Could you check a few things on this model? Use its own coordinates, in mm. A direction names the side the tool comes from. Coordinates: 2 decimals unless noted, no trailing zeros. Loops run counter-clockwise (first coordinate to the right, second up) from the corner with the lowest first, then second, coordinate; pieces in that order, holes last. Notation, with made-up numbers: (85.25, 44.5) - (95.25, 44.5) arc R28 ccw to (95.25, 80.5) - close; hole circle Ø10 at (86.5, 54). An arc over 180 degrees is marked (long way). One line per item, written item: value. Start each with the question number.
(1) On a 3-axis mill with a long thin cutter (end or side, diameter ignored), from which of +Z, -Z, +X, -X, +Y, -Y can I reach the whole of each face in a straight line? I mean faces 4 (the face through (-12, 2, 16)), 5 (the face through (-12, -2, 8.271)), 6 (the face through (-13.5, -38.1, 13.662)), 7 (the face through (-17, -4.65, 12)), 8 (the face through (-17, 5, 13.662)). Say none if no direction works.
(2) If we section it at D-D on x = -15.75: Write out the boundary of the cut face in (y, z) (3 decimals), then the cut area to 3 significant figures.
(3) I'm going to push flat-ended pins straight in: P1, Ø3, axis at x = -12.5, z = 6.5, coming from the +Y side; P2, Ø4, axis at x = -14.5, z = 10, coming from the -Y side; P3, Ø4, axis at x = -10.5, y = -15, coming from the +Z side. Where does each tip first touch, or does it pass through?
(4) If we section it at A-A on z = 15: Write out the boundary of the cut face in (x, y), then the cut area to 3 significant figures.
(5) If I drill on line 1 along Y through (x, z) = (-17, 9.25); line 2 along Y through (x, z) = (-12.5, 16.75); line 3 along Y through (x, z) = (-14.25, 11.75), over which ranges is the centre line in solid material (lowest first)? Write a range as from..to.
(6) If we section it at B-B on x = -13: Write out the boundary of the cut face in (y, z) (3 decimals), then the cut area to 3 significant figures.
(7) If we section it at C-C on y = -37.05: Write out the boundary of the cut face in (x, z).
(8) If we mould it in two halves opening along Y, with no side actions, what happens to faces 1 (the face through (-10.488, -2, 15)), 2 (the face through (-15, -16, 1.162)), 3 (the face through (-15, 0, 7))? For each: pulls with the +Y half, pulls with the -Y half, needs draft (parallel to the pull), parting line crosses it, or undercut.
```python
from build123d import *

# Parameters (mm, degrees)
ESBO_O1_W                = 13.25
ESBO_O1_H                = 12.5
RESSALTO_EXTRUS_O1_DEPTH = 4.65
ESBO_O2_W                = 13.25
ESBO_O2_H                = 32.05
RESSALTO_EXTRUS_O2_DEPTH = 5
ESBO_O3_W                = 13.25
ESBO_O3_H                = 4.65
RESSALTO_EXTRUS_O3_DEPTH = 12.5
ESBO_O4_W                = 13.25
ESBO_O4_H                = 5
RESSALTO_EXTRUS_O4_DEPTH = 10
ESBO_O5_W                = 13.25
ESBO_O5_H                = 5
RESSALTO_EXTRUS_O5_DEPTH = 10
ESBO_O6_R                = 1.5
CORTE_EXTRUS_O1_DEPTH    = 10
ESBO_O7_R                = 1
CORTE_EXTRUS_O2_DEPTH    = 14.25
ESBO_O8_R                = 1
CORTE_EXTRUS_O3_DEPTH    = 14.25
ESBO_O9_W                = 3
ESBO_O9_H                = 10.390977072
CORTE_EXTRUS_O4_DEPTH    = 10
ESBO_O10_W               = 3
ESBO_O10_H               = 2
CORTE_EXTRUS_O5_DEPTH    = 10


with BuildPart() as part:
    # Esboço1 → Ressalto-extrusão1 (new body)
    with BuildSketch(Plane(origin=(0, 0, 0), x_dir=(1, 0, 0), z_dir=(0, 1, 0))):
        with Locations((-15.112918198, -12.411797698)):
            Rectangle(ESBO_O1_W, ESBO_O1_H)
    extrude(amount=-RESSALTO_EXTRUS_O1_DEPTH)

    # Esboço2 → Ressalto-extrusão2 (add)
    with BuildSketch(Plane(origin=(0, 0, 6.161797698), x_dir=(-1, 0, 0), z_dir=(0, 0, -1))):
        with Locations((15.112918198, -16.025)):
            Rectangle(ESBO_O2_W, ESBO_O2_H)
    extrude(amount=RESSALTO_EXTRUS_O2_DEPTH)

    # Esboço3 → Ressalto-extrusão3 (add)
    with BuildSketch(Plane.XY.offset(6.161797698)):
        with Locations((-15.112918198, -29.725)):
            Rectangle(ESBO_O3_W, ESBO_O3_H)
    extrude(amount=RESSALTO_EXTRUS_O3_DEPTH)

    # Esboço4 → Ressalto-extrusão4 (add)
    with BuildSketch(Plane(origin=(0, -32.05, 0), x_dir=(-1, 0, 0), z_dir=(0, -1, 0))):
        with Locations((15.112918198, -16.161797698)):
            Rectangle(ESBO_O4_W, ESBO_O4_H)
    extrude(amount=RESSALTO_EXTRUS_O4_DEPTH)

    # Esboço5 → Ressalto-extrusão5 (add)
    with BuildSketch(Plane(origin=(0, 0, 0), x_dir=(1, 0, 0), z_dir=(0, 1, 0))):
        with Locations((-15.112918198, -16.161797698)):
            Rectangle(ESBO_O5_W, ESBO_O5_H)
    extrude(amount=RESSALTO_EXTRUS_O5_DEPTH)

    # Esboço6 → Corte-extrusão1 (cut)
    with BuildSketch(Plane(origin=(0, 0, 13.661797698), x_dir=(-1, 0, 0), z_dir=(0, 0, -1))):
        with Locations((15.112918198, 5)):
            Circle(ESBO_O6_R)
        with Locations((15.112918198, -37.05)):
            Circle(ESBO_O6_R)
    extrude(amount=-CORTE_EXTRUS_O1_DEPTH, mode=Mode.SUBTRACT)

    # Esboço7 → Corte-extrusão2 (cut, through all)
    with BuildSketch(Plane(origin=(-8.487918198, 0, 0), x_dir=(0, 0, -1), z_dir=(1, 0, 0))):
        with Locations((-12.411797698, -2.325)):
            Circle(ESBO_O7_R)
    extrude(amount=-CORTE_EXTRUS_O2_DEPTH, mode=Mode.SUBTRACT)

    # Esboço8 → Corte-extrusão3 (cut, through all)
    with BuildSketch(Plane(origin=(-8.487918198, 0, 0), x_dir=(0, 0, -1), z_dir=(1, 0, 0))):
        with Locations((-12.411797698, -29.725)):
            Circle(ESBO_O8_R)
    extrude(amount=-CORTE_EXTRUS_O3_DEPTH, mode=Mode.SUBTRACT)

    # Esboço9 → Corte-extrusão4 (cut)
    with BuildSketch(Plane(origin=(0, 0, 0), x_dir=(1, 0, 0), z_dir=(0, 1, 0))):
        with Locations((-11.987918198, -13.466309162)):
            Rectangle(ESBO_O9_W, ESBO_O9_H)
    extrude(amount=-CORTE_EXTRUS_O4_DEPTH, mode=Mode.SUBTRACT)

    # Esboço10 → Corte-extrusão5 (cut)
    with BuildSketch(Plane(origin=(0, 0, 13.661797698), x_dir=(-1, 0, 0), z_dir=(0, 0, -1))):
        with Locations((11.987918198, 1)):
            Rectangle(ESBO_O10_W, ESBO_O10_H)
    extrude(amount=-CORTE_EXTRUS_O5_DEPTH, mode=Mode.SUBTRACT)


solid = part.part
```
Values:
1. face 4: +Z, -Z
1. face 5: +Z, +Y
1. face 6: -Z, +X, -X, -Y
1. face 7: +Z, +X, -X
1. face 8: -Z, +X, -X, +Y
2. outline: (-42.05, 13.662) - (-38.408, 13.662) - (-38.408, 18.662) - (-42.05, 18.662) - close; (-35.692, 13.662) - (-32.05, 13.662) - (-32.05, 1.162) - (0, 1.162) - (0, 13.662) - (3.642, 13.662) - (3.642, 18.662) - (-4.65, 18.662) - (-4.65, 6.162) - (-27.4, 6.162) - (-27.4, 18.662) - (-35.692, 18.662) - close; (6.358, 13.662) - (10, 13.662) - (10, 18.662) - (6.358, 18.662) - close; hole circle Ø2 at (-29.725, 12.412); hole circle Ø2 at (-2.325, 12.412)
2. area: 343 mm2
3. P1: stops at y = 0
3. P2: stops at y = -32.05
3. P3: stops at z = 6.16
4. outline: (-21.74, -42.05) - (-8.49, -42.05) - (-8.49, -27.4) - (-21.74, -27.4) - close; (-21.74, -4.65) - (-13.49, -4.65) - (-13.49, 2) - (-10.49, 2) - (-10.49, -4.65) - (-8.49, -4.65) - (-8.49, 10) - (-21.74, 10) - close; hole circle Ø3 at (-15.11, -37.05); hole circle Ø3 at (-15.11, 5)
4. area: 354 mm2
5. line 1: y = -32.05..-27.4, -4.65..0
5. line 2: y = -42.05..-27.4, 2..10
5. line 3: y = -32.05..-30.47, -28.98..-27.4, -4.65..-3.07, -1.58..0
6. outline: (-42.05, 13.662) - (-32.05, 13.662) - (-32.05, 1.162) - (0, 1.162) - (0, 8.271) - (-4.65, 8.271) - (-4.65, 6.162) - (-27.4, 6.162) - (-27.4, 18.662) - (-42.05, 18.662) - close; (2, 13.662) - (10, 13.662) - (10, 18.662) - (2, 18.662) - close; hole circle Ø2 at (-29.725, 12.412)
6. area: 315 mm2
7. outline: (-21.74, 13.66) - (-16.61, 13.66) - (-16.61, 18.66) - (-21.74, 18.66) - close; (-13.61, 13.66) - (-8.49, 13.66) - (-8.49, 18.66) - (-13.61, 18.66) - close
8. face 1: undercut
8. face 2: needs draft
8. face 3: pulls with the +Y half
